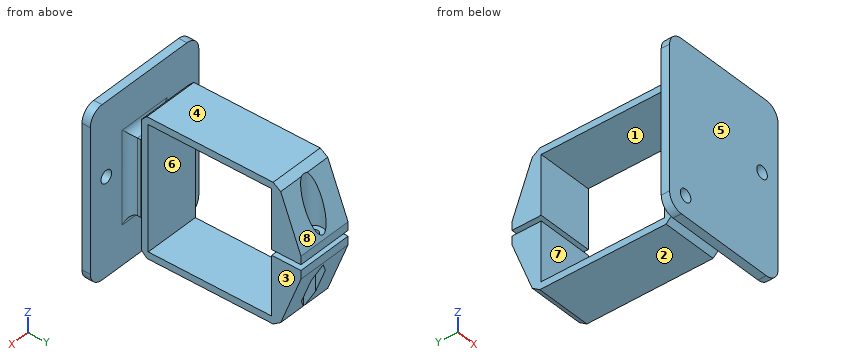
Solid Edge part; units mm, degrees
sketch "Sketch1" plane through (0, 0, 0) normal (0, -1, 0) x (1, 0, 0)
  circle A0 centre (16.25, 4.37) radius 2.25
  circle A1 centre (-16.25, -23.13) radius 2.25
  line L0 (-23.05, -30.5) -> (23.05, -30.5)
  line L1 (23.05, -30.5) -> (23.05, 30.5)
  line L2 (23.05, 30.5) -> (-23.05, 30.5)
  line L3 (-23.05, 30.5) -> (-23.05, -30.5)
  dimension "D1" = 23.05
  dimension "D2" = 16.25
  dimension "D3" = 16.25
extrude "Protrusion1" add sketch "Sketch1" against normal blind 3
fillet "Redondeo_2" radius 5 4 edges at (23.05, 1.5, 30.5) (-23.05, 1.5, 30.5) (23.05, 1.5, -30.5) (-23.05, 1.5, -30.5)
sketch "Sketch2" plane through (0, 3, 0) normal (0, 1, 0) x (-1, 0, 0)
  line L0 (-6.5, 13.5) -> (6.5, 13.5)
  line L1 (6.5, 13.5) -> (6.5, -13.5)
  line L2 (6.5, -13.5) -> (-6.5, -13.5)
  line L3 (-6.5, -13.5) -> (-6.5, 13.5)
extrude "ProtrusiónExtruida_4" add sketch "Sketch2" along normal blind 6
sketch "Sketch3" plane through (8.5, 6, 0) normal (1, 0, 0) x (0, 1, 0)
  line L0 (49.8, -22.15) -> (5.5, -22.15)
  line L1 (5.5, -22.15) -> (5.5, 22.15)
  line L2 (5.5, 22.15) -> (49.8, 22.15)
  line L3 (49.8, 22.15) -> (49.8, -22.15)
  line L4 (52.3, -24.65) -> (3, -24.65)
  line L5 (3, -24.65) -> (3, 24.65)
  line L6 (3, 24.65) -> (52.3, 24.65)
  line L7 (52.3, 24.65) -> (52.3, -24.65)
  dimension "D1" = 49.8
extrude "ProtrusiónExtruida_5" add sketch "Sketch3" against normal blind 20
sketch "Sketch4" plane through (8.5, 33.65, 0) normal (1, 0, 0) x (0, 1, 0)
  line L0 (29.65, -1) -> (19.65, -1)
  line L1 (19.65, -1) -> (19.65, 1)
  line L2 (19.65, 1) -> (29.65, 1)
  line L3 (29.65, 1) -> (29.65, -1)
  dimension "D1" = 29.65
extrude "VaciadoExtruido_1" cut sketch "Sketch4" against normal blind 43.1103
sketch "Sketch5" plane through (8.5, 33.65, 0) normal (1, 0, 0) x (0, 1, 0)
  line L0 (24.65, -24.65) -> (24.65, -1)
  line L1 (24.65, -1) -> (32.65, -1)
  line L2 (32.65, -1) -> (32.65, -4)
  line L3 (32.65, -4) -> (24.65, -24.65)
  line L4 (24.65, 1) -> (32.65, 1)
  line L5 (32.65, 1) -> (32.65, 4)
  line L6 (24.65, 24.65) -> (32.65, 4)
  line L7 (24.65, 24.65) -> (24.65, 1)
  dimension "D1" = 24.65
  dimension "D2" = 32.65
extrude "v_20" add sketch "Sketch5" against normal blind 20
sketch "Sketch6" plane through (-1.5, 33.65, 24.65) normal (0, 0, 1) x (0, 1, 0)
  circle A0 centre (28.65, 0) radius 1.75
extrude "VaciadoExtruido_2" cut sketch "Sketch6" against normal blind 71.0094
sketch "Sketch7" plane through (-1.5, 33.65, 24.65) normal (0, 0, 1) x (0, 1, 0)
  circle A0 centre (28.65, 0) radius 3.5
extrude "Cutout1" cut sketch "Sketch7" against normal up to vertex (20.65 mm away)
chamfer "Chaflán_2" distance 2 angle 45 4 edges at (-1.5, 58.3, 24.65) (-1.5, 9, 24.65) (-1.5, 58.3, -24.65) (-1.5, 9, -24.65)
sketch "Sketch8" plane through (-1.5, 33.65, -24.65) normal (0, 0, -1) x (0, -1, 0)
  line L0 (-32.15, 0) -> (-30.4, 3.0311)
  line L1 (-30.4, 3.0311) -> (-26.9, 3.0311)
  line L2 (-26.9, 3.0311) -> (-25.15, 0)
  line L3 (-25.15, 0) -> (-26.9, -3.0311)
  line L4 (-26.9, -3.0311) -> (-30.4, -3.0311)
  line L5 (-30.4, -3.0311) -> (-32.15, 0)
extrude "Cutout2" cut sketch "Sketch8" against normal up to vertex (20.65 mm away)
fillet "Redondeo_3" radius 3 4 edges at (6.5, 3, 0) (0, 3, 13.5) (0, 3, -13.5) (-6.5, 3, 0)
fillet "Redondeo_4" radius 2 4 edges at (0, 9, -13.5) (-6.5, 9, 0) (0, 9, 13.5) (6.5, 9, 0)
CAD build for the part. Positions are in the model's coordinates, mm. Face numbers are marked on the shaded views. A direction names the side the tool comes from. Coordinates: 2 decimals unless noted, no trailing zeros. Write each loop counter-clockwise with the first axis right and the second up, starting at its lowest first coordinate (ties: lowest second). Pieces come first, ordered by that corner, then holes. Notation, with made-up numbers: (87.25, -27.5) -> (112.25, -27.5) arc R12 ccw to (112.25, -6.5) -> close; hole circle Ø5 at (-11.5, 64.25). An arc over 180 degrees is marked (long way). Return JSON: item names as keys, results as strings. Group by question number.
Q1. Which spindle directions (+Z, -Z, +X, -X, +Y, -Y) get a long thin tool onto all of the face, cutting with end or side? Do the marked faces 1, 2, 3 and 4. Say none if no direction does.
Q2. Drill centre lines: line 1 (Z direction, x = -3, y = 20.5); line 2 (Z direction, x = 16.25, y = 0.65); line 3 (X direction, y = 62.3, z = 2.3). Where is each one in solid material? Low to high.
Q3. Cut at B-B, the plane y = 30.5. Give the cut face in (x, z).
Q4. Pull direction Z, two halves, no side cores. Call the marked faces 5, 6, 7 and 8: released by +Z, released by -Z, zero draft, split by the parting line, or undercut.
Q5. Cut at C-C, the plane z = 19. Give the cut face in (x, y).
Q6. Flat gauge pins, fed straight in: pin 1 (5 mm diameter, centred on x = 3.5, y = 24.5, fed in from -Z); pin 2 (3 mm diameter, centred on y = 56.5, z = -18, fed in from +X); pin 3 (4 mm diameter, centred on y = 61.5, z = -8, fed in from -X); pin 4 (5 mm diameter, centred on x = 13, z = -19.5, fed in from -Y). Where does each tip first touch, or does it go through?
Q7. Cut at D-D, the plane y = 62.5. Give the cut face in (x, z), then the cut area to 3 significant figures.
Q8. Cut at A-A, the plane x = 16.25. Give the cut face in (y, z), then the cut area to 4 significant figures.
Returned:
{
 "1": {"face 1": "+X, -X", "face 2": "-Z, +X, -X, +Y", "face 3": "+Z, -Z, +X, +Y", "face 4": "+Z, +X, -X, +Y"},
 "2": {"line 1": "z = -24.65 to -22.15, 22.15 to 24.65", "line 2": "z = -30.5 to 2.12, 6.62 to 30.5", "line 3": "x = -11.5 to -3.25, 0.25 to 8.5"},
 "3": {"outline": "(-11.5, -24.65) -> (8.5, -24.65) -> (8.5, -22.15) -> (-11.5, -22.15) -> close; (-11.5, 22.15) -> (8.5, 22.15) -> (8.5, 24.65) -> (-11.5, 24.65) -> close"},
 "4": {"face 5": "zero draft", "face 6": "undercut", "face 7": "undercut", "face 8": "released by +Z"},
 "5": {"outline": "(-23.05, 0) -> (23.05, 0) -> (23.05, 3) -> (-23.05, 3) -> close; (-11.5, 9) -> (8.5, 9) -> (8.5, 11.5) -> (-11.5, 11.5) -> close; (-11.5, 55.8) -> (8.5, 55.8) -> (8.5, 60.49) -> (1.49, 60.49) arc R3.5 cw to (-4.49, 60.49) -> (-11.5, 60.49) -> close"},
 "6": {"pin 1": "stops at z = -24.65", "pin 2": "stops at x = 8.5", "pin 3": "stops at x = -11.5", "pin 4": "stops at y = 0"},
 "7": {"outline": "(-11.5, -13.81) -> (-4.53, -13.81) -> (-4.53, -4) -> (-3.24, -4) -> (-3.24, -1) -> (-11.5, -1) -> close; (-11.5, 1) -> (-3.24, 1) -> (-3.24, 4) -> (-4.99, 4) -> (-4.99, 13.81) -> (-11.5, 13.81) -> close; (0.24, -4) -> (1.53, -4) -> (1.53, -13.81) -> (8.5, -13.81) -> (8.5, -1) -> (0.24, -1) -> close; (0.24, 1) -> (8.5, 1) -> (8.5, 13.81) -> (1.99, 13.81) -> (1.99, 4) -> (0.24, 4) -> close", "area": "363 mm2"},
 "8": {"outline": "(0, -30.5) -> (3, -30.5) -> (3, 2.12) -> (0, 2.12) -> close; (0, 6.62) -> (3, 6.62) -> (3, 30.5) -> (0, 30.5) -> close", "area": "169.5 mm2"}
}
